Check sheet for the modelled part. Datum: model origin and axes. Units: mm. Round coordinates to 2 decimals unless told otherwise and drop trailing zeros. Loops run counter-clockwise (first coordinate to the right, second up) from the corner with the lowest first, then second, coordinate; pieces in that order, holes last. Notation, with made-up numbers: (20.25, 7.5) - (47.25, 7.5) arc R23 ccw to (47.25, 19.5) - close; hole circle Ø5 at (-34.75, -3.5). An arc over 180 degrees is marked (long way). Put each result on its own line as item: value.
```python
from build123d import *

# Parameters (mm, degrees)
F0_R     = 1.5875
F1_DEPTH = 9.525
F2_SIZE  = 0.127
F3_SIZE  = 0.127


with BuildPart() as f1:
    # F0 (on Right) → F1 (new body)
    with BuildSketch(Plane.YZ):
        Circle(F0_R)
    extrude(amount=F1_DEPTH)

    # F2
    f2_edges = [f1.edges().sort_by_distance(p)[0] for p in [
        (9.525, -1.5875, 0),
    ]]
    chamfer(f2_edges, length=F2_SIZE)

    # F3
    f3_edges = [f1.edges().sort_by_distance(p)[0] for p in [
        (0, -1.5875, 0),
    ]]
    chamfer(f3_edges, length=F3_SIZE)


solid = f1.part
```
Item 1: Release check for a two-part mould opening along Z. For faces 1 (the flat face through (0, 0, 0)), 2 (the cylindrical face through (4.7, -0.34, -1.55)) record: +Z half, -Z half, draft (parallel to the pull), parting line (faces both ways), or undercut.
Filled sheet:
face 1: draft
face 2: parting line
Item 2: Section check A-A on x = 3. Enter the section's corners in (y, z) (1 decimal).
Filled sheet:
outline: circle Ø3.2 at (0, 0)
Item 3: Thickness scan on line 1 (Z direction, x = 7.25, y = -0.45); line 2 (Y direction, x = 6, z = 0.4); line 3 (Y direction, x = 5.25, z = 1.4). Record the ranges inside material, lowest first. Write a range as from..to.
Filled sheet:
line 1: -1.52..1.52
line 2: -1.54..1.54
line 3: -0.75..0.75
Item 4: Go/stop test with a flat-tipped pin: pin 1 (1.5 mm diameter, centred on x = 6, z = -0.5, fed in from -Y). Record where the tip stops, or that it passes through.
Filled sheet:
pin 1: y = -1.59
